Source: CAD feature listing. Evaluate the final solid. Frame: model axes, mm. A direction names the side the tool comes from. Give positions to 0.01 mm unless a question says otherwise; leave off trailing zeros. Write each loop counter-clockwise with the first axis right and the second up, starting at its lowest first coordinate (ties: lowest second). Pieces come first, ordered by that corner, then holes.
```python
from build123d import *

# Parameters (mm, degrees)
SKETCH1_R           = 1.3890625
SKETCH1_R_2         = 1.905
BOSS_EXTRUDE1_DEPTH = 6.35


with BuildPart() as part:
    # Sketch1 → Boss-Extrude1 (new body)
    with BuildSketch(Plane.XY):
        with BuildLine():
            Line((-12.7, 0), (12.7, 0))
            Line((12.7, 0), (12.7, -44.17993629))
            Line((12.7, -44.17993629), (25.4, -44.17993629))
            Line((25.4, -44.17993629), (25.4, -23.822954819))
            add(Edge.make_bspline(
                [(44.901870562, 9.48833089), (22.852171125, -3.715928222), (25.4, -23.822954819)],
                knots=[5.247063621, 5.247063621, 5.247063621, 6.283185307, 6.283185307, 6.283185307], degree=2, weights=[1, 0.868781076, 1]))
            ThreePointArc((44.901870562, 9.48833089), (46.747333824, 17.526669162), (38.641141335, 19.046623163))
            ThreePointArc((38.641141335, 19.046623163), (0, 6.664444687), (-38.641141335, 19.046623163))
            ThreePointArc((-38.641141335, 19.046623163), (-46.747333824, 17.526669162), (-44.901870562, 9.48833089))
            add(Edge.make_bspline(
                [(-25.4, -23.822954819), (-22.852171125, -3.715928222), (-44.901870562, 9.48833089)],
                knots=[0, 0, 0, 1.036121686, 1.036121686, 1.036121686], degree=2, weights=[1, 0.868781076, 1]))
            Line((-25.4, -23.822954819), (-25.4, -44.17993629))
            Line((-25.4, -44.17993629), (-12.7, -44.17993629))
            Line((-12.7, -44.17993629), (-12.7, 0))
        make_face()
        with Locations(Location((41.964300524, 14.393758438, 0), (0, 0, 180))):
            Circle(SKETCH1_R, mode=Mode.SUBTRACT)
        with Locations((-41.964300524, 14.393758438)):
            Circle(SKETCH1_R, mode=Mode.SUBTRACT)
        with Locations((-19.05, -17.78)):
            Circle(SKETCH1_R_2, mode=Mode.SUBTRACT)
        with Locations((-19.05, -36.83)):
            Circle(SKETCH1_R_2, mode=Mode.SUBTRACT)
        with Locations(Location((19.05, -36.83, 0), (0, 0, 180))):
            Circle(SKETCH1_R_2, mode=Mode.SUBTRACT)
        with Locations(Location((19.05, -17.78, 0), (0, 0, 180))):
            Circle(SKETCH1_R_2, mode=Mode.SUBTRACT)
    extrude(amount=BOSS_EXTRUDE1_DEPTH)


solid = part.part
```
1. Access query for faces 1 (the cylindrical face through (0.577, 6.667, 3.131)), 2 (the cylindrical face through (-43.352, 14.455, 3.131)), 3 (the flat face through (0, 0, 3)), 4 (the flat face through (25.4, -34, 3)), 5 (the flat face through (-25.4, -34, 3)). Directions: +Z, -Z, +X, -X, +Y, -Y. A direction counts if a zero-diameter tool reaches every point of the face in a straight line with its end or side. Return the directions, or none.
2. Section query B-B (x = -20). Return loops of the section in (y, z), plus the area to 3 significant figures.
3. Section query D-D (z = 1.25). Give the number of separate pieces and of enclosed holes in the cut face, plus the area to 3 significant figures.
4. Pin query (flat end, axial travel): P1, Ø1.9, axis at y = -16.5, z = 2, coming from the +X side; P2, Ø1.5, axis at y = -10, z = 1.5, coming from the +X side; P3, Ø1.5, axis at x = 36.5, z = 4.5, coming from the +Y side. Return the tip coordinate at first contact, or that it passes through.
5. Line query: probe 1 along Y at (x, z) = (-19.5, 5); probe 2 along Y at (x, z) = (19.05, 2.5) (3 decimals); probe 3 along X at (y, z) = (-16.5, 5). Output: solid intervals per line, ascending.
6. Pull-direction query (Y, two-part tool) for faces 6 (the cylindrical face through (46.817, 17.418, 3.131)), 7 (the flat face through (12.7, -22, 3)), 8 (the cylindrical face through (42.988, 13.455, 3.131)); classes: pulls with the +Y half, pulls with the -Y half, needs draft (parallel to the pull), parting line crosses it, or undercut.
7. Section query C-C (x = 19.05). Return loops of the section in (y, z) (3 decimals).
8. Section query A-A (y = -36.83). Return loops of the section in (x, z) (3 decimals), plus the area to 3 significant figures.
The answers:
1. face 1: +Z, -Z, +Y
1. face 2: +Z, -Z
1. face 3: +Z, -Z, -Y
1. face 4: +Z, -Z, +X, -Y
1. face 5: +Z, -Z, -X, -Y
2. outline: (-44.18, 0) - (-38.48, 0) - (-38.48, 6.35) - (-44.18, 6.35) - close; (-35.18, 0) - (-19.43, 0) - (-19.43, 6.35) - (-35.18, 6.35) - close; (-16.13, 0) - (9.74, 0) - (9.74, 6.35) - (-16.13, 6.35) - close
2. area: 300 mm2
3. separate pieces: 1
3. enclosed holes: 6
3. area: 2,150 mm2
4. P1: stops at x = 25.65
4. P2: stops at x = 27.57
4. P3: stops at y = 18.08
5. probe 1: y = -44.18 to -38.68, -34.98 to -19.63, -15.93 to 9.59
5. probe 2: y = -44.18 to -38.735, -34.925 to -19.685, -15.875 to 9.452
5. probe 3: x = -25.49 to -20.46, -17.64 to -12.7, 12.7 to 17.64, 20.46 to 25.49
6. face 6: parting line crosses it
6. face 7: needs draft
6. face 8: undercut
7. outline: (-44.18, 0) - (-38.735, 0) - (-38.735, 6.35) - (-44.18, 6.35) - close; (-34.925, 0) - (-19.685, 0) - (-19.685, 6.35) - (-34.925, 6.35) - close; (-15.875, 0) - (9.452, 0) - (9.452, 6.35) - (-15.875, 6.35) - close
8. outline: (-25.4, 0) - (-20.955, 0) - (-20.955, 6.35) - (-25.4, 6.35) - close; (-17.145, 0) - (-12.7, 0) - (-12.7, 6.35) - (-17.145, 6.35) - close; (12.7, 0) - (17.145, 0) - (17.145, 6.35) - (12.7, 6.35) - close; (20.955, 0) - (25.4, 0) - (25.4, 6.35) - (20.955, 6.35) - close
8. area: 113 mm2
